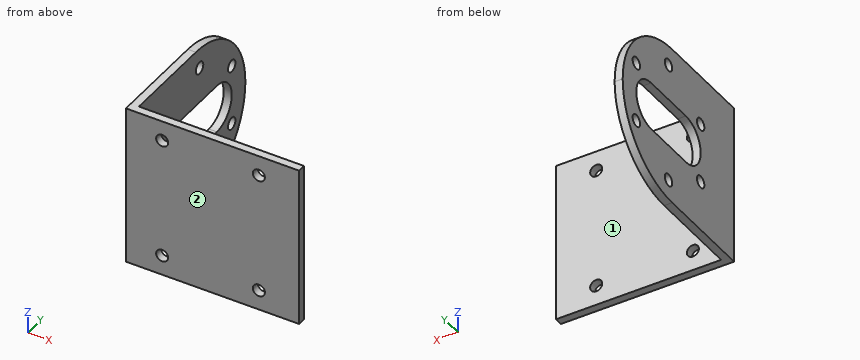
```python
from build123d import *

# Parameters (mm, degrees)
EXTRUDE_1_DEPTH     = 40
SKETCH_2_R          = 1.5
CUT_EXTRUDE_1_DEPTH = 73.78736154
FILLET_1_R          = 20
CUT_EXTRUDE_2_DEPTH = 73.78736154
SKETCH_4_R          = 1.5
CUT_EXTRUDE_3_DEPTH = 72.624018318


with BuildPart() as part:
    # 草图1 → 拉伸-薄壁1 (new body)
    with BuildSketch(Plane.XY):
        Polygon((41, 0), (0, 0), (0, 43), (-2, 43), (-2, -2), (41, -2), align=None)
    extrude(amount=EXTRUDE_1_DEPTH)

    # 草图2 → 切除-拉伸1 (cut, through all)
    with BuildSketch(Plane.ZY.offset(2)):
        with Locations((35, 24.5)):
            Circle(SKETCH_2_R)
        with Locations((27.5, 11.509618943)):
            Circle(SKETCH_2_R)
        with Locations((12.5, 11.509618943)):
            Circle(SKETCH_2_R)
        with Locations((5, 24.5)):
            Circle(SKETCH_2_R)
        with Locations((12.5, 37.490381057)):
            Circle(SKETCH_2_R)
        with Locations((27.5, 37.490381057)):
            Circle(SKETCH_2_R)
    extrude(amount=-CUT_EXTRUDE_1_DEPTH, mode=Mode.SUBTRACT)

    # 圆角1
    fillet_1_edges = [part.edges().sort_by_distance(p)[0] for p in [
        (-1, 43, 40),
        (-1, 43, 0),
    ]]
    fillet(fillet_1_edges, radius=FILLET_1_R - 0.0001)  # a hair under: the kernel refuses the full size

    # 草图3 → 切除-拉伸2 (cut, through all)
    with BuildSketch(Plane.ZY.offset(2)):
        with BuildLine():
            Line((26, 31.5), (26, 17.5))
            ThreePointArc((26, 17.5), (20, 11.5), (14, 17.5))
            Line((14, 17.5), (14, 31.5))
            ThreePointArc((14, 31.5), (20, 37.5), (26, 31.5))
        make_face()
    extrude(amount=-CUT_EXTRUDE_2_DEPTH, mode=Mode.SUBTRACT)

    # 草图4 → 切除-拉伸3 (cut, through all)
    with BuildSketch(Plane(origin=(0, 0, 0), x_dir=(1, 0, 0), z_dir=(0, 1, 0))):
        with Locations(Location((7, -35, 0), (0, 0, 270))):
            Circle(SKETCH_4_R)
        with Locations(Location((31, -35, 0), (0, 0, 270))):
            Circle(SKETCH_4_R)
        with Locations(Location((31, -5, 0), (0, 0, 270))):
            Circle(SKETCH_4_R)
        with Locations(Location((7, -5, 0), (0, 0, 270))):
            Circle(SKETCH_4_R)
    extrude(amount=-CUT_EXTRUDE_3_DEPTH, mode=Mode.SUBTRACT)


solid = part.part
```
The listing builds one solid part. Answer for the finished solid, in the listing's coordinates (mm). Face numbers are marked on the shaded views. A direction names the side the tool comes from. Coordinates: 2 decimals unless noted, no trailing zeros. Write each loop counter-clockwise with the first axis right and the second up, starting at its lowest first coordinate (ties: lowest second). Pieces come first, ordered by that corner, then holes. Notation, with made-up numbers: (19, -11) - (39, -11) arc R16 ccw to (39, -5) - close; hole circle Ø8 at (86.25, 65.5). An arc over 180 degrees is marked (long way). Return JSON: item names as keys, results as strings. Group by question number.
Q1. The part is cut by section A-A on y = 19. Write down the section's boundary in (x, z), and give its area (3 significant figures).
Q2. The part is cut by section C-C on y = 24.5. Write down the section's boundary in (x, z), and give its area (3 significant figures).
Q3. The part is cut by section B-B on x = 7. Write down the section's boundary in (y, z), and give its area (3 significant figures).
Q4. Which of the six approach directions +Z, -Z, +X, -X, +Y, -Y give full straight-line access (tool end or side, diameter ignored) to the marked faces 1 and 2?
Q5. Find the intervals of material crossed by line 1 along Y through (x, z) = (-1, 27); line 2 along Y through (x, z) = (-1.05, 27.5); line 3 along X through (y, z) = (3, 6), in increasing order. Write a range as [from, to].
Q6. Flat-ended cylindrical pins translate along their axes: pin 1 Ø0.6 at (x, y) = (-1.5, 27) entering from -Z; pin 2 Ø4 at (y, z) = (24.5, 5) entering from +X; pin 3 Ø20 at (x, z) = (19.5, 25.5) entering from +Y. Find the tip coordinate at first contact, or state that the pin passes through.
Q7. The part is cut by section D-D on z = 27.5. Write down the section's boundary in (x, y).
Evaluation:
{
 "1": {"outline": "(-2, 0) - (0, 0) - (0, 14) - (-2, 14) - close; (-2, 26) - (0, 26) - (0, 40) - (-2, 40) - close", "area": "56.0 mm2"},
 "2": {"outline": "(-2, 0.06) - (0, 0.06) - (0, 3.5) - (-2, 3.5) - close; (-2, 6.5) - (0, 6.5) - (0, 14) - (-2, 14) - close; (-2, 26) - (0, 26) - (0, 33.5) - (-2, 33.5) - close; (-2, 36.5) - (0, 36.5) - (0, 39.94) - (-2, 39.94) - close", "area": "43.8 mm2"},
 "3": {"outline": "(-2, 0) - (0, 0) - (0, 3.5) - (-2, 3.5) - close; (-2, 6.5) - (0, 6.5) - (0, 33.5) - (-2, 33.5) - close; (-2, 36.5) - (0, 36.5) - (0, 40) - (-2, 40) - close", "area": "68.0 mm2"},
 "4": {"face 1": "+Z, -Z, +X, +Y", "face 2": "+Z, -Z, +X, -X, -Y"},
 "5": {"line 1": "y = [-2, 10.1], [12.92, 36.08], [38.9, 41.74]", "line 2": "y = [-2, 10.01], [13.01, 35.99], [38.99, 41.54]", "line 3": "x = [-2, 0]"},
 "6": {"pin 1": "stops at z = 0.35", "pin 2": "stops at x = 0", "pin 3": "stops at y = 0"},
 "7": {"outline": "(-2, -2) - (41, -2) - (41, 0) - (0, 0) - (0, 10.01) - (-2, 10.01) - close; (-2, 13.01) - (0, 13.01) - (0, 35.99) - (-2, 35.99) - close; (-2, 38.99) - (0, 38.99) - (0, 41.54) - (-2, 41.54) - close"}
}
